Work out the finished part from the listing and answer in its coordinate system (mm). Coordinates: 2 decimals unless noted, no trailing zeros. Write each loop counter-clockwise with the first axis right and the second up, starting at its lowest first coordinate (ties: lowest second). Pieces come first, ordered by that corner, then holes. Notation, with made-up numbers: (83, -23) - (109, -23) arc R15 cw to (109, -8) - close; hole circle Ø11 at (22.5, -11). An arc over 180 degrees is marked (long way). One line per item, written item: value.
```python
from build123d import *

# Parameters (mm, degrees)
F0_R     = 12.7
F1_DEPTH = 50.8


with BuildPart() as f1:
    # F0 (on Top) → F1 (new body)
    with BuildSketch(Plane.XY):
        Polygon((-76.2, 0), (0, 0), (0, 25.4), (-38.1, 50.8), (-76.2, 50.8), align=None)
        with Locations((-38.1, 25.4)):
            Circle(F0_R, mode=Mode.SUBTRACT)
    extrude(amount=F1_DEPTH)


solid = f1.part
```
Item 1: Consider probe 1 along Y at (x, z) = (-38.1, 33); probe 2 along X at (y, z) = (25, 15); probe 3 along Y at (x, z) = (-38, 23). Determine where each line is inside the solid, lowest interval first.
Evaluation:
probe 1: y = 0 to 12.7, 38.1 to 50.8
probe 2: x = -76.2 to -50.79, -25.41 to 0
probe 3: y = 0 to 12.7, 38.1 to 50.73
Item 2: Section A-A, the plane z = 37 is taken. Determine the outline of the cut face in (x, y).
Evaluation:
outline: (-76.2, 0) - (0, 0) - (0, 25.4) - (-38.1, 50.8) - (-76.2, 50.8) - close; hole circle Ø25.4 at (-38.1, 25.4)
Item 3: Section D-D, the plane x = -23 is taken. Determine the outline of the cut face in (y, z).
Evaluation:
outline: (0, 0) - (40.73, 0) - (40.73, 50.8) - (0, 50.8) - close
Item 4: Section B-B, the plane y = 15 is taken. Determine the outline of the cut face in (x, z).
Evaluation:
outline: (-76.2, 0) - (-45.39, 0) - (-45.39, 50.8) - (-76.2, 50.8) - close; (-30.81, 0) - (0, 0) - (0, 50.8) - (-30.81, 50.8) - close
Item 5: Determine the mould class of faces 1 (the face through (-57, 50.8, 25)), 2 (the face through (-47, 14, 50.8)), 3 (the face through (-39.753, 37.992, 25.044)) for opening direction Y: +Y half, -Y half, draft (parallel to the pull), parting line (faces both ways), or undercut.
Evaluation:
face 1: +Y half
face 2: draft
face 3: undercut
Item 6: Section C-C, the plane y = 20.5 is taken. Determine the outline of the cut face in (x, z), then the cut area to 3 significant figures.
Evaluation:
outline: (-76.2, 0) - (-49.82, 0) - (-49.82, 50.8) - (-76.2, 50.8) - close; (-26.38, 0) - (0, 0) - (0, 50.8) - (-26.38, 50.8) - close
area: 2,680 mm2
Item 7: Given pin 1 (8 mm diameter, centred on x = -46.5, y = 25, fed in from +Z), flat-ended and moving along its own axis, determine where the tip first touches the part or whether it passes through.
Evaluation:
pin 1: passes through
